```python
from build123d import *

# Parameters (mm, degrees)
BOSS_EXTRUDE1_DEPTH = 35
SKETCH2_W           = 17.696874766
SKETCH2_H           = 12.5
BOSS_EXTRUDE2_DEPTH = 17.5
BOSS_EXTRUDE3_REACH = 59.1
SKETCH3_W           = 17.576942212
SKETCH3_H           = 12.5
SKETCH6_R           = 5
CUT_EXTRUDE4_DEPTH  = 34.153314003
CUT_EXTRUDE5_START  = -10.195
SKETCH7_R           = 22.5
CUT_EXTRUDE5_DEPTH  = 10.195
CUT_EXTRUDE6_START  = -10.195
CUT_EXTRUDE6_DEPTH  = 10.195
FILLET1_R           = 10


with BuildPart() as part:
    # Sketch1 → Boss-Extrude1 (new body)
    with BuildSketch(Plane(origin=(0, 0, 0), x_dir=(1, 0, 0), z_dir=(0, 1, 0))):
        with BuildLine():
            Line((-23.500000002, -12.2928564), (-23.500000002, -17.153314003))
            Line((-23.500000002, -17.153314003), (41.499999998, -17.153314003))
            Line((41.499999998, -17.153314003), (41.499999998, -12.153314003))
            ThreePointArc((41.499999998, -12.153314003), (29.653468029, -11.155125098), (23.999999998, -0.696874766))
            Line((23.999999998, -0.696874766), (23.999999998, 17))
            Line((23.999999998, 17), (0.15591238, 17))
            ThreePointArc((0.15591238, 17), (-7.603392609, -0.932132231), (-23.500000002, -12.2928564))
        make_face()
    extrude(amount=BOSS_EXTRUDE1_DEPTH)

    # Sketch2 → Boss-Extrude2 (add)
    with BuildSketch(Plane(origin=(23.999999998, 0, 0), x_dir=(0, 0, -1), z_dir=(1, 0, 0))):
        with Locations((8.151562617, 28.75)):
            Rectangle(SKETCH2_W, SKETCH2_H)
    extrude(amount=BOSS_EXTRUDE2_DEPTH)

    # Sketch3 → Boss-Extrude3 (add, up to next)
    with BuildSketch(Plane.XY.offset(0.696874766), mode=Mode.PRIVATE) as boss_extrude3_sk1:
        with Locations((32.711528892, 28.75)):
            Rectangle(SKETCH3_W, SKETCH3_H)
    boss_extrude3_tool1 = extrude(boss_extrude3_sk1.sketch, amount=BOSS_EXTRUDE3_REACH, mode=Mode.PRIVATE) - part.part
    add(boss_extrude3_tool1.solids().sort_by_distance((32.711529, 28.75, 0.696875))[0])

    # Sketch6 → Cut-Extrude4 (cut)
    with BuildSketch(Plane(origin=(0, 0, -17), x_dir=(-1, 0, 0), z_dir=(0, 0, -1))):
        with Locations((5.34408762, 7.5)):
            Circle(SKETCH6_R)
        with Locations((5.34408762, 27.5)):
            Circle(SKETCH6_R)
    extrude(amount=-CUT_EXTRUDE4_DEPTH, mode=Mode.SUBTRACT)

    # Sketch7 → Cut-Extrude5 (cut)
    with BuildSketch(Plane.XZ.offset(CUT_EXTRUDE5_START)):
        with Locations((36.499999998, 0.696874766)):
            Circle(SKETCH7_R)
    extrude(amount=CUT_EXTRUDE5_DEPTH, mode=Mode.SUBTRACT)

    # Sketch8 → Cut-Extrude6 (cut)
    with BuildSketch(Plane.XZ.offset(CUT_EXTRUDE6_START)):
        with BuildLine():
            Line((-4.500000002, 17.153314003), (41.499999998, 17.153314003))
            Line((41.499999998, 17.153314003), (41.499999998, -17))
            Line((41.499999998, -17), (22.605014445, -17))
            Line((22.605014445, -17), (14.020220559, -0.256810916))
            ThreePointArc((14.020220559, -0.256810916), (8.209356978, 12.117427379), (-4.500000002, 17.153314003))
        make_face()
    extrude(amount=CUT_EXTRUDE6_DEPTH, mode=Mode.SUBTRACT)

    # Fillet1
    fillet1_edges = [part.edges().sort_by_distance(p)[0] for p in [
        (41.499999998, 22.5975, 17.153314003),
    ]]
    fillet(fillet1_edges, radius=FILLET1_R)


solid = part.part
```
Source: CAD feature listing. Evaluate the final solid. Frame: model axes, mm. A direction names the side the tool comes from. Give positions to 0.01 mm unless a question says otherwise; leave off trailing zeros. Loops run counter-clockwise (first coordinate to the right, second up) from the corner with the lowest first, then second, coordinate; pieces in that order, holes last. Notation, with made-up numbers: (-16.5, -37) -> (22.5, -37) arc R26 ccw to (22.5, -9) -> close; hole circle Ø7 at (73.25, 60.5). An arc over 180 degrees is marked (long way). Use a Markdown table: item, result. Add a question column.
(1) Pull-direction query (X, two-part tool) for faces 1 (the face through (16, 21, -17)), 2 (the face through (-0.35, 7.72, 4.73)), 3 (the face through (29.038, 16.261, 10.725)), 4 (the face through (41.5, 29, -5)); classes: +X half, -X half, draft (parallel to the pull), parting line (faces both ways), or undercut.
(2) Ray query, line 1 (Y direction, x = -9.5, z = 11.5); line 2 (Z direction, x = -7, y = 14); line 3 (X direction, y = 24, z = 10). Return the intervals inside material, ascending.
(3) Section query A-A (y = 25.5). Output: boundary loops of the cut face in (x, z), then the cut area to 3 significant figures.
(4) Section query B-B (z = 6). Output: boundary loops of the cut face in (x, y) (3 decimals).
(5) First-contact query: pin 1 Ø9 at (x, y) = (-5.34, 27.5) entering from -Z; pin 2 Ø19 at (x, z) = (36.5, -8) entering from -Y; pin 3 Ø1.5 at (y, z) = (8, -2) entering from -X; pin 4 Ø3 at (y, z) = (7.5, 10) entering from +X. Flat tips, straight axial feed; report the tip coordinate or a pass-through.
(6) Section query D-D (z = -9). Output: boundary loops of the cut face in (x, y) (3 decimals), then the cut area to 3 significant figures.
(7) Section query C-C (x = 33). Output: boundary loops of the cut face in (y, z) (3 decimals).
(8) Access query for faces 5 (the face through (-23.5, 17, 15)), 6 (the face through (24, 16, -8)), 7 (the face through (8.351, 5.169, 11.982)). Directions: +Z, -Z, +X, -X, +Y, -Y. A direction counts if a zero-diameter tool reaches every point of the face in a straight line with its end or side. Return the directions, or none.
Checked values:
| question | item | result |
|---|---|---|
| 1 | face 1 | draft |
| 1 | face 2 | undercut |
| 1 | face 3 | undercut |
| 1 | face 4 | +X half |
| 2 | line 1 | 0 to 4.72, 10.28 to 24.72, 30.28 to 35 |
| 2 | line 2 | 0.16 to 17.15 |
| 2 | line 3 | -18.44 to -8.91, -1.77 to 41.09 |
| 3 | outline | (-23.5, 12.29) arc R36.5 cw to (-9.93, 3.54) -> (-9.93, 17.15) -> (-23.5, 17.15) -> close; (-0.76, -12.49) arc R36.5 cw to (0.16, -17) -> (41.5, -17) -> (41.5, 7.15) arc R10 ccw to (31.5, 17.15) -> (-0.76, 17.15) -> close |
| 3 | area | 1,540 mm^2 |
| 4 | outline | (-12.585, 0) -> (12.515, 0) -> (12.515, 10.195) -> (25.181, 10.195) -> (25.181, 22.5) -> (41.5, 22.5) -> (41.5, 35) -> (-12.585, 35) -> close; hole circle Ø10 at (-5.344, 7.5); hole circle Ø10 at (-5.344, 27.5) |
| 5 | pin 1 | through |
| 5 | pin 2 | y = 22.5 |
| 5 | pin 3 | x = -0.5 |
| 5 | pin 4 | x = 11.19 |
| 6 | outline | (-1.894, 0) -> (16.197, 0) -> (16.197, 10.195) -> (24, 10.195) -> (24, 22.5) -> (41.5, 22.5) -> (41.5, 35) -> (-1.894, 35) -> (-1.894, 31.119) arc R5 cw to (-1.894, 23.881) -> (-1.894, 11.119) arc R5 cw to (-1.894, 3.881) -> close |
| 6 | area | 1,030 mm^2 |
| 7 | outline | (10.195, 12.697) -> (22.5, 12.697) -> (22.5, -17) -> (35, -17) -> (35, 17.04) -> (10.195, 17.04) -> close |
| 8 | face 5 | +Z, -Z, -X, +Y, -Y |
| 8 | face 6 | -Z, +X, -Y |
| 8 | face 7 | +Z, +X, -Y |
